Can you work these out from the model? Positions are in its coordinate system, mm. A direction names the side the tool comes from. Coordinates: 2 decimals unless noted, no trailing zeros. Loops run counter-clockwise (first coordinate to the right, second up) from the corner with the lowest first, then second, coordinate; pieces in that order, holes last.
```python
from build123d import *

# Parameters (mm, degrees)
SKETCH1_W           = 26.67
SKETCH1_H           = 20.32
BOSS_EXTRUDE1_DEPTH = 3.175
SKETCH2_R           = 1.905
SKETCH2_R_2         = 1.397
BOSS_EXTRUDE2_DEPTH = 6.35
FILLET1_R           = 1


with BuildPart() as part:
    # Sketch1 → Boss-Extrude1 (new body)
    with BuildSketch(Plane(origin=(0, 0, 0), x_dir=(1, 0, 0), z_dir=(0, 1, 0))):
        with Locations((-10.451352941, 1.434352941)):
            Rectangle(SKETCH1_W, SKETCH1_H)
    extrude(amount=BOSS_EXTRUDE1_DEPTH)

    # Sketch2 → Boss-Extrude2 (add)
    with BuildSketch(Plane(origin=(0, 3.175, 0), x_dir=(1, 0, 0), z_dir=(0, 1, 0))):
        with Locations((-21.246352941, 9.054352941)):
            Circle(SKETCH2_R)
        with Locations((-21.246352941, 9.054352941)):
            Circle(SKETCH2_R_2, mode=Mode.SUBTRACT)
        with Locations((0.343647059, 9.054352941)):
            Circle(SKETCH2_R)
        with Locations((0.343647059, 9.054352941)):
            Circle(SKETCH2_R_2, mode=Mode.SUBTRACT)
        with Locations((0.343647059, -6.185647059)):
            Circle(SKETCH2_R)
        with Locations((0.343647059, -6.185647059)):
            Circle(SKETCH2_R_2, mode=Mode.SUBTRACT)
        with Locations((-21.246352941, -6.185647059)):
            Circle(SKETCH2_R)
        with Locations((-21.246352941, -6.185647059)):
            Circle(SKETCH2_R_2, mode=Mode.SUBTRACT)
    extrude(amount=BOSS_EXTRUDE2_DEPTH)

    # Fillet1
    fillet1_edges = [part.edges().sort_by_distance(p)[0] for p in [
        (-23.786352941, 1.5875, -11.594352941),
        (2.883647059, 1.5875, -11.594352941),
        (2.883647059, 1.5875, 8.725647059),
        (-23.786352941, 1.5875, 8.725647059),
    ]]
    fillet(fillet1_edges, radius=FILLET1_R)


solid = part.part
```
Item 1: Suppose I cut it at A-A, the plane y = 8. Please give me the cut outline in (x, z) (3 decimals).
Results are:
outline: circle Ø3.81 at (-21.246, -9.054); circle Ø3.81 at (-21.246, 6.186); circle Ø3.81 at (0.344, -9.054); circle Ø3.81 at (0.344, 6.186); hole circle Ø2.794 at (-21.246, -9.054); hole circle Ø2.794 at (-21.246, 6.186); hole circle Ø2.794 at (0.344, -9.054); hole circle Ø2.794 at (0.344, 6.186)
Item 2: I need wall thicknesses on line 1 along X through (y, z) = (7.75, 7); line 2 along X through (y, z) = (9.25, 6.5); line 3 along Y through (x, z) = (-3.75, 5) (3 decimals). Which ranges of each line are inside material? Lowest first, please.
Results are:
line 1: x = -22.97 to -22.38, -20.11 to -19.52, -1.38 to -0.79, 1.48 to 2.07
line 2: x = -23.13 to -22.61, -19.89 to -19.37, -1.54 to -1.02, 1.7 to 2.22
line 3: y = 0 to 3.175
Item 3: We'd pull the mould along X, two halves only. Please class faces 3 (the face through (2.884, 2, -1)), 4 (the face through (-11, 0, -2)), 5 (the face through (0, 3.175, 6)): +X half, -X half, draft (parallel to the pull), parting line (faces both ways), or undercut.
Results are:
face 3: +X half
face 4: draft
face 5: undercut
Item 4: On a 3-axis mill with a long thin cutter (end or side, diameter ignored), from which of +Z, -Z, +X, -X, +Y, -Y can I reach the whole of each face in a straight line? I mean faces 1 (the face through (-23.501, 1.61, 8.425)), 2 (the face through (-0.686, 6.306, 5.241)). Say none if no direction works.
Results are:
face 1: +Z, -X, +Y, -Y
face 2: +Y
Item 5: I'm going to push flat-ended pins straight in: P1, Ø3, axis at y = 7, z = 5.5, coming from the -X side; P2, Ø0.8, axis at x = -21, z = 6, coming from the +Y side (3 decimals). Where does each tip first touch, or does it pass through?
Results are:
P1: stops at x = -23.15
P2: stops at y = 3.175
Item 6: Suppose I cut it at C-C, the plane z = -4.25. Please give me the cut outline in (x, y) (3 decimals).
Results are:
outline: (-23.786, 0) - (2.884, 0) - (2.884, 3.175) - (-23.786, 3.175) - close
Item 7: Suppose I cut it at B-B, the plane x = 1.25. Please give me the cut outline in (y, z) (3 decimals).
Results are:
outline: (0, -11.594) - (3.175, -11.594) - (3.175, -10.73) - (9.525, -10.73) - (9.525, -10.117) - (3.175, -10.117) - (3.175, -7.991) - (9.525, -7.991) - (9.525, -7.379) - (3.175, -7.379) - (3.175, 4.51) - (9.525, 4.51) - (9.525, 5.123) - (3.175, 5.123) - (3.175, 7.249) - (9.525, 7.249) - (9.525, 7.861) - (3.175, 7.861) - (3.175, 8.726) - (0, 8.726) - close
Item 8: Suppose I cut it at D-D, the plane x = -4. Please give me the cut outline in (y, z) (3 decimals).
Results are:
outline: (0, -11.594) - (3.175, -11.594) - (3.175, 8.726) - (0, 8.726) - close
